The figure shows three views and two pictorial views of one solid part (mm, origin at its lowest corner). Answer the questions. Round coordinates to 2 decimals unless told otherwise and drop trailing zeros. Order: outer loops, then holes, each group sorted by start corner. A loop starts at its lowest first (then second) coordinate and runs counter-clockwise, first axis right, second up. Notation, with made-up numbers: (-2, 77) - (24, 77) arc R17 cw to (24, 89) - close; hole circle Ø11 at (9.25, 67.25). An arc over 180 degrees is marked (long way). Answer as a JSON object with one key per item and string values. Group by question number.
Q1. A cutting plane is placed at D-D on z = 29. Determine the outline of the cut face in (x, y).
Q2. A cutting plane is placed at C-C on x = 17.2. Determine the outline of the cut face in (y, z).
Q3. Given pin 1 Ø1.6 at (y, z) = (3, 49.5) entering from +X; pin 2 Ø1.6 at (x, y) = (86, 3) entering from -Z; pin 3 Ø1 at (x, z) = (19.5, 43) entering from +Y, each flat-ended and moving along its own axis, determine where each tip first touches the part or whether it passes through.
Q4. A cutting plane is placed at A-A on y = 3.4. Determine the outline of the cut face in (x, z), and give its area (3 significant figures).
Q5. A cutting plane is placed at B-B on z = 36.7. Determine the outline of the cut face in (x, y), and give its area (3 significant figures).
Q6. Consider line 1 (X direction, y = 1.4, z = 36.7); line 2 (Z direction, x = 17.5, y = 0.25); line 3 (Y direction, x = 41, z = 48). Determine where each line is inside the solid, lowest interval first.
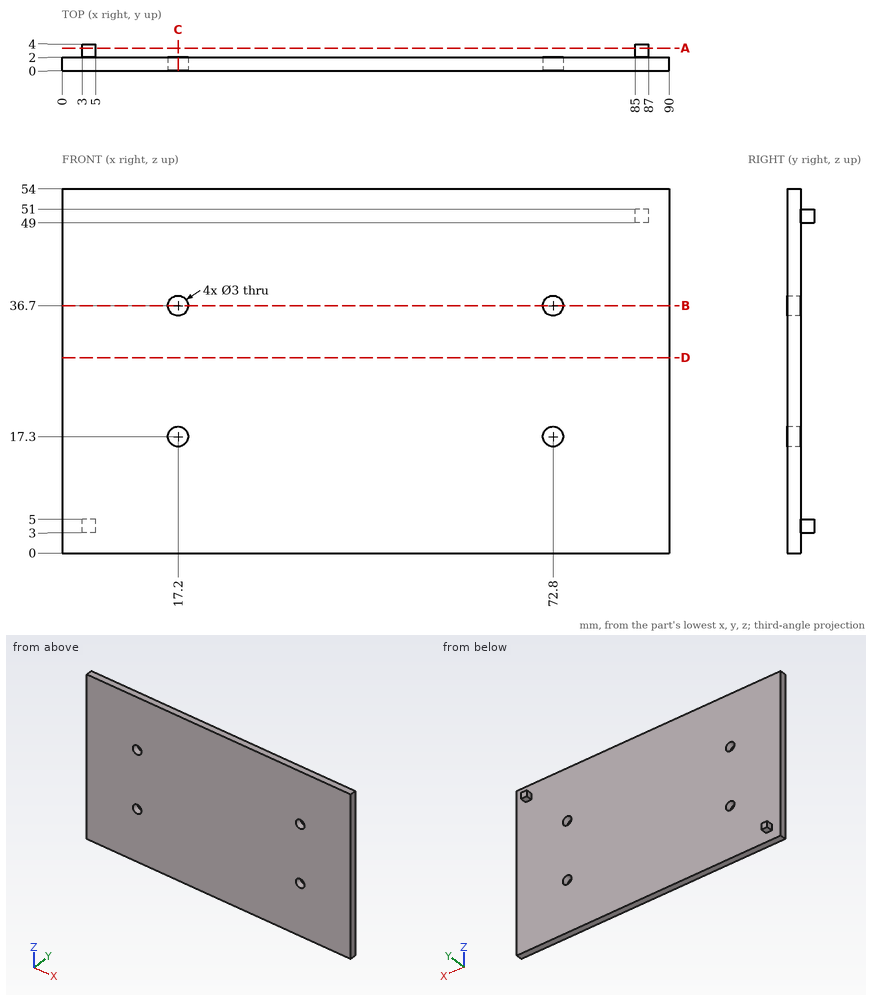
Result set:
{
 "1": {"outline": "(0, 0) - (90, 0) - (90, 2) - (0, 2) - close"},
 "2": {"outline": "(0, 0) - (2, 0) - (2, 15.8) - (0, 15.8) - close; (0, 18.8) - (2, 18.8) - (2, 35.2) - (0, 35.2) - close; (0, 38.2) - (2, 38.2) - (2, 54) - (0, 54) - close"},
 "3": {"pin 1": "stops at x = 87", "pin 2": "stops at z = 49", "pin 3": "stops at y = 2"},
 "4": {"outline": "(3, 3) - (5, 3) - (5, 5) - (3, 5) - close; (85, 49) - (87, 49) - (87, 51) - (85, 51) - close", "area": "8.00 mm²"},
 "5": {"outline": "(0, 0) - (15.7, 0) - (15.7, 2) - (0, 2) - close; (18.7, 0) - (71.3, 0) - (71.3, 2) - (18.7, 2) - close; (74.3, 0) - (90, 0) - (90, 2) - (74.3, 2) - close", "area": "168 mm²"},
 "6": {"line 1": "x = 0 to 15.7, 18.7 to 71.3, 74.3 to 90", "line 2": "z = 0 to 15.83, 18.77 to 35.23, 38.17 to 54", "line 3": "y = 0 to 2"}
}
